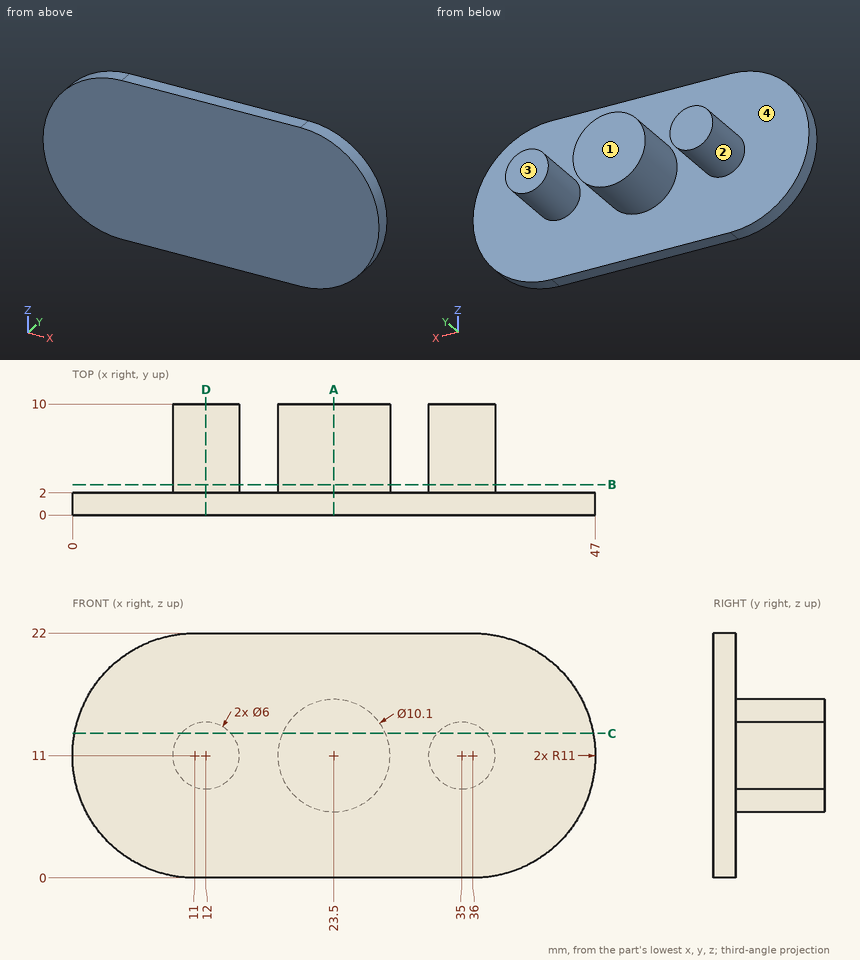
Check sheet for the drawn part. Datum: minimum x, y, z corner. Units: mm. A direction names the side the tool comes from. Round coordinates to 2 decimals unless told otherwise and drop trailing zeros. Loops run counter-clockwise (first coordinate to the right, second up) from the corner with the lowest first, then second, coordinate; pieces in that order, holes last. Notation, with made-up numbers: (66.5, 69) - (84.5, 69) arc R21 ccw to (84.5, 103) - close; hole circle Ø7 at (-25, -29.5). An arc over 180 degrees is marked (long way). Write each question's results on one line, items separated by ' | '. Start each with the question number.
Q1. Cross-section at D-D on x = 12. Enter the section's corners in (y, z), and give its area (3 significant figures).
Q2. Gauge pin test, flat ends, axial feed: P1, Ø12, axis at x = 28, z = 15, coming from the +Y side; P2, Ø2, axis at x = 5.5, z = 5, coming from the +Y side; P3, Ø4, axis at x = 26.5, y = 6, coming from the -Z side. Record the tip position at first contact, or that the pin passes through.
Q3. Release check for a two-part mould opening along X. For the marked faces 1 and 2 record: +X half, -X half, draft (parallel to the pull), parting line (faces both ways), or undercut.
Q4. Cross-section at C-C on z = 13. Enter the section's corners in (x, y), and give its area (3 significant figures).
Q5. Cross-section at B-B on y = 2.75. Enter the section's corners in (x, z).
Q6. Access from +Z, -Z, +X, -X, +Y, -Y to the whole of each face (thin tool, end or side, straight path). Record for the marked faces 3 and 4.
Q7. Thickness scan on line 1 (X direction, y = 8, z = 13.5); line 2 (Y direction, x = 39.5, z = 18.5); line 3 (Z direction, x = 14, y = 8.5). Record the ranges inside material, lowest first. Write a range as [from, to].
Q8. Cross-section at A-A on x = 23.5. Enter the section's corners in (y, z), and give its area (3 significant figures).
Answers below:
1) outline: (0, 0) - (2, 0) - (2, 8) - (10, 8) - (10, 14) - (2, 14) - (2, 22) - (0, 22) - close | area: 92.0 mm²
2) P1: stops at y = 10 | P2: stops at y = 2 | P3: stops at z = 6.05
3) face 1: draft | face 2: undercut
4) outline: (0.18, 0) - (46.82, 0) - (46.82, 2) - (37.24, 2) - (37.24, 10) - (32.76, 10) - (32.76, 2) - (28.14, 2) - (28.14, 10) - (18.86, 10) - (18.86, 2) - (14.24, 2) - (14.24, 10) - (9.76, 10) - (9.76, 2) - (0.18, 2) - close | area: 239 mm²
5) outline: circle Ø6 at (12, 11); circle Ø10.1 at (23.5, 11); circle Ø6 at (35, 11)
6) face 3: +Z, -Z, +X, -X, +Y | face 4: +Y
7) line 1: x = [10.34, 13.66], [19.11, 27.89], [33.34, 36.66] | line 2: y = [0, 2] | line 3: z = [8.76, 13.24]
8) outline: (0, 0) - (2, 0) - (2, 5.95) - (10, 5.95) - (10, 16.05) - (2, 16.05) - (2, 22) - (0, 22) - close | area: 125 mm²
